CAD build for the part. Positions are in the model's coordinates, mm. Coordinates: 2 decimals unless noted, no trailing zeros. Order: outer loops, then holes, each group sorted by start corner. A loop starts at its lowest first (then second) coordinate and runs counter-clockwise, first axis right, second up. Notation, with made-up numbers: M 54.25,38 L 91.25,38 A24 cw 91.25,66 Z; hole C 55,24 d7. An arc over 180 degrees is marked long. One line per item, written item: value.
from build123d import *

# Parameters (mm, degrees)
BOSS_EXTRUDE1_DEPTH = 3
SKETCH5_R           = 1.8
CUT_EXTRUDE2_DEPTH  = 106.270616959
CUT_EXTRUDE3_DEPTH  = 106.270616959


with BuildPart() as part:
    # Sketch2 → Boss-Extrude1 (new body)
    with BuildSketch(Plane(origin=(0, 0, 0), x_dir=(1, 0, 0), z_dir=(0, 1, 0))):
        with BuildLine():
            Line((-42, 17), (-42, -17))
            Line((-42, -17), (-72.784271247, -47.784271247))
            Line((-72.784271247, -47.784271247), (-60.284271247, -60.284271247))
            Line((-60.284271247, -60.284271247), (-32, -32))
            Line((-32, -32), (32, -32))
            Line((32, -32), (60.284271247, -60.284271247))
            Line((60.284271247, -60.284271247), (72.784271247, -47.784271247))
            Line((72.784271247, -47.784271247), (42, -17))
            Line((42, -17), (42, 17))
            Line((42, 17), (72.784271247, 47.784271247))
            ThreePointArc((72.784271247, 47.784271247), (0, 75.995741025), (-72.784271247, 47.784271247))
            Line((-72.784271247, 47.784271247), (-42, 17))
        make_face()
    extrude(amount=BOSS_EXTRUDE1_DEPTH)

    # Sketch5 → Cut-Extrude2 (cut, through all)
    with BuildSketch(Plane(origin=(0, 3, 0), x_dir=(1, 0, 0), z_dir=(0, 1, 0))):
        with Locations(Location((-57.5, 43.25, 0), (0, 0, 270))):
            Circle(SKETCH5_R)
        with Locations(Location((56, 43.25, 0), (0, 0, 270))):
            Circle(SKETCH5_R)
        with Locations(Location((56.75, -43.25, 0), (0, 0, 270))):
            Circle(SKETCH5_R)
        with Locations(Location((-56.75, -43.25, 0), (0, 0, 270))):
            Circle(SKETCH5_R)
    extrude(amount=-CUT_EXTRUDE2_DEPTH, mode=Mode.SUBTRACT)

    # Sketch6 → Cut-Extrude3 (cut, through all)
    with BuildSketch(Plane(origin=(0, 3, 0), x_dir=(1, 0, 0), z_dir=(0, 1, 0))):
        Polygon((-38, 14.077369669), (-3, 14.077369669), (-3, 6.077369669), align=None)
        Polygon((-38, 11), (-3, 3), (-38, 3), align=None)
        Polygon((-3, -14.077369669), (-3, -6.077369669), (-38, -14.077369669), align=None)
        Polygon((-3, -3), (-38, -3), (-38, -11), align=None)
        Polygon((38, -14.077369669), (3, -14.077369669), (3, -6.077369669), align=None)
        Polygon((38, -11), (3, -3), (38, -3), align=None)
        Polygon((3, 3), (38, 3), (38, 11), align=None)
        Polygon((3, 14.077369669), (3, 6.077369669), (38, 14.077369669), align=None)
        Polygon((-38, -17), (-3, -17), (-3, -27), align=None)
        Polygon((3, -17), (3, -27), (38, -17), align=None)
    extrude(amount=-CUT_EXTRUDE3_DEPTH, mode=Mode.SUBTRACT)


solid = part.part
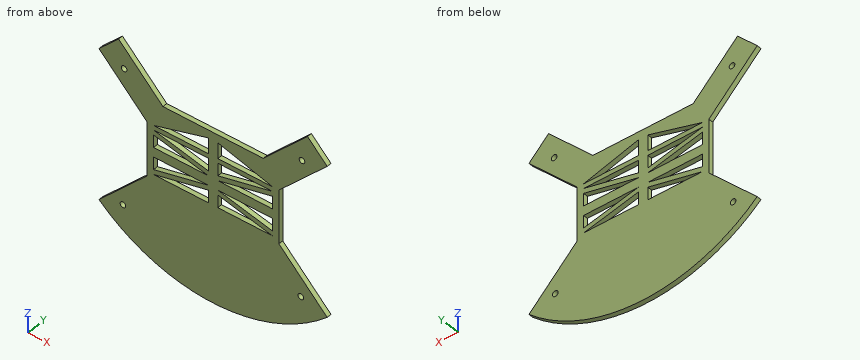
Q1. Slice it at A-A (z = 35). List the corners of the cut face in (x, y).
Recorded:
outline: M -60,0 L -35,0 L -35,3 L -60,3 Z; M 35,0 L 60,0 L 60,3 L 35,3 Z
Q2. Slice it at B-B (x = -51). List the corners of the cut face in (y, z).
Recorded:
outline: M 0,-63.19 L 3,-63.19 L 3,-26 L 0,-26 Z; M 0,26 L 3,26 L 3,51 L 0,51 Z
Q3. Slice it at C-C (y = 2.3). Give the number of separate pieces and of enclosed holes in the cut face, plus the area to 3 significant figures.
Recorded:
separate pieces: 1
enclosed holes: 14
area: 10,300 mm^2
Q4. Slice it at D-D (z = -8). List the corners of the cut face in (x, y) (1 decimal).
Recorded:
outline: M -42,0 L -38,0 L -38,3 L -42,3 Z; M -24.9,0 L -11.4,0 L -11.4,3 L -24.9,3 Z; M -3,0 L 3,0 L 3,3 L -3,3 Z; M 11.4,0 L 24.9,0 L 24.9,3 L 11.4,3 Z; M 38,0 L 42,0 L 42,3 L 38,3 Z
Q5. Drill centre lines: line 1 along Z through (x, y) = (-17, 1.9); line 2 along X through (y, z) = (2.05, -43.25); line 3 along Z through (x, y) = (58, 1.2). Where is each one in solid material? Low to high.
Recorded:
line 1: z = -74.65 to -14.08, -9.28 to -6.2, -3 to 3, 6.2 to 9.28, 14.08 to 17, 23 to 32
line 2: x = -68.25 to -59.3, -55.7 to 54.2, 57.8 to 68.25
line 3: z = -59.1 to -33, 33 to 41.95, 44.55 to 58
Q6. Pin check, flat tips, straight feed: pin 1 Ø0.9 at (y, z) = (1.5, 24) entering from +X; pin 2 Ø1.5 at (y, z) = (2, 8.5) entering from +X; pin 3 Ø1.5 at (x, y) = (-27, 2) entering from -Z. Stop position of each tip, or through.
Recorded:
pin 1: stops at x = 49.45
pin 2: stops at x = 42
pin 3: stops at z = -72.76
